Part model, mm, in its own coordinate system. A direction names the side the tool comes from. Round coordinates to 2 decimals unless told otherwise and drop trailing zeros. Loops run counter-clockwise (first coordinate to the right, second up) from the corner with the lowest first, then second, coordinate; pieces in that order, holes last.
from build123d import *

# Parameters (mm, degrees)
SKETCH1_R           = 1.5
BOSS_EXTRUDE2_DEPTH = 3.8
BOSS_EXTRUDE3_START = -3.8
SKETCH2_W           = 3.5
SKETCH2_H           = 7
SKETCH2_H_2         = 5.25
BOSS_EXTRUDE3_DEPTH = 3.8
CUT_EXTRUDE1_DEPTH  = 2.3
SKETCH4_W           = 3.5
SKETCH4_H           = 7
CUT_EXTRUDE2_DEPTH  = 1.5
FILLET1_R           = 4


with BuildPart() as part:
    # Sketch1 → Boss-Extrude2 (new body)
    # profile 1 of 5: a face of its own
    with BuildSketch(Plane(origin=(0, 0, 0), x_dir=(1, 0, 0), z_dir=(0, 1, 0))):
        with BuildLine():
            Line((-11.834936491, -1.25), (-11.834936491, 1.25))
            ThreePointArc((-11.834936491, 1.25), (-16.5, 0), (-11.834936491, -1.25))
        make_face()
        with Locations(Location((-14, 0, 0), (0, 0, 90))):
            Circle(SKETCH1_R, mode=Mode.SUBTRACT)
    # profile 2 of 5: a face of its own
    with BuildSketch(Plane(origin=(0, 0, 0), x_dir=(1, 0, 0), z_dir=(0, 1, 0))):
        with BuildLine():
            ThreePointArc((-11.5, 0), (-11.585185434, 0.647047613), (-11.834936491, 1.25))
            Line((-11.834936491, 1.25), (-11.834936491, -1.25))
            ThreePointArc((-11.834936491, -1.25), (-11.585185434, -0.647047613), (-11.5, 0))
        make_face()
    # profile 3 of 5: a face of its own
    with BuildSketch(Plane(origin=(0, 0, 0), x_dir=(1, 0, 0), z_dir=(0, 1, 0))):
        with BuildLine():
            Line((11.834936491, 1.25), (-11.834936491, 1.25))
            ThreePointArc((-11.834936491, 1.25), (-11.585185434, 0.647047613), (-11.5, 0))
            ThreePointArc((-11.5, 0), (-11.585185434, -0.647047613), (-11.834936491, -1.25))
            Line((-11.834936491, -1.25), (11.834936491, -1.25))
            ThreePointArc((11.834936491, -1.25), (11.5, 0), (11.834936491, 1.25))
        make_face()
    # profile 4 of 5: a face of its own
    with BuildSketch(Plane(origin=(0, 0, 0), x_dir=(1, 0, 0), z_dir=(0, 1, 0))):
        with BuildLine():
            Line((11.834936491, -1.25), (11.834936491, 1.25))
            ThreePointArc((11.834936491, 1.25), (11.5, 0), (11.834936491, -1.25))
        make_face()
    # profile 5 of 5: a face of its own
    with BuildSketch(Plane(origin=(0, 0, 0), x_dir=(1, 0, 0), z_dir=(0, 1, 0))):
        with BuildLine():
            ThreePointArc((16.5, 0), (14.647047613, 2.414814566), (11.834936491, 1.25))
            Line((11.834936491, 1.25), (11.834936491, -1.25))
            ThreePointArc((11.834936491, -1.25), (14.647047613, -2.414814566), (16.5, 0))
        make_face()
        with Locations(Location((14, 0, 0), (0, 0, 90))):
            Circle(SKETCH1_R, mode=Mode.SUBTRACT)
    extrude(amount=BOSS_EXTRUDE2_DEPTH)

    # Sketch2 → Boss-Extrude3 (add)
    with BuildSketch(Plane(origin=(0, 3.8, 0), x_dir=(1, 0, 0), z_dir=(0, 1, 0)).offset(BOSS_EXTRUDE3_START)):
        with Locations((-10.5, 10)):
            Rectangle(SKETCH2_W, SKETCH2_H)
        with BuildLine():
            Line((-8.75, 6.5), (-12.25, 6.5))
            Line((-12.25, 6.5), (-12.25, 1.785357107))
            ThreePointArc((-12.25, 1.785357107), (-12.024251438, 1.531802083), (-11.834936491, 1.25))
            Line((-11.834936491, 1.25), (-8.75, 1.25))
            Line((-8.75, 1.25), (-8.75, 6.5))
        make_face()
        with Locations((10.5, -3.875)):
            Rectangle(SKETCH2_W, SKETCH2_H_2)
        with Locations((10.5, -10)):
            Rectangle(SKETCH2_W, SKETCH2_H)
    extrude(amount=BOSS_EXTRUDE3_DEPTH)

    # Sketch3 → Cut-Extrude1 (cut)
    with BuildSketch(Plane.XZ):
        with BuildLine():
            Line((11.834936491, 1.25), (8.75, 1.25))
            Line((8.75, 1.25), (-11.834936491, 1.25))
            ThreePointArc((-11.834936491, 1.25), (-11.585185434, 0.647047613), (-11.5, 0))
            ThreePointArc((-11.5, 0), (-11.585185434, -0.647047613), (-11.834936491, -1.25))
            Line((-11.834936491, -1.25), (-8.75, -1.25))
            Line((-8.75, -1.25), (11.834936491, -1.25))
            ThreePointArc((11.834936491, -1.25), (11.5, 0), (11.834936491, 1.25))
        make_face()
        with BuildLine():
            Line((12.25, 6.5), (8.75, 6.5))
            Line((8.75, 6.5), (8.75, 1.25))
            Line((8.75, 1.25), (11.834936491, 1.25))
            ThreePointArc((11.834936491, 1.25), (12.024251438, 1.531802083), (12.25, 1.785357107))
            Line((12.25, 1.785357107), (12.25, 6.5))
        make_face()
        with BuildLine():
            ThreePointArc((-11.834936491, -1.25), (-12.024251438, -1.531802083), (-12.25, -1.785357107))
            Line((-12.25, -1.785357107), (-12.25, -6.5))
            Line((-12.25, -6.5), (-8.75, -6.5))
            Line((-8.75, -6.5), (-8.75, -1.25))
            Line((-8.75, -1.25), (-11.834936491, -1.25))
        make_face()
    extrude(amount=-CUT_EXTRUDE1_DEPTH, mode=Mode.SUBTRACT)

    # Sketch4 → Cut-Extrude2 (cut)
    with BuildSketch(Plane.XZ):
        with Locations((-10.5, -10)):
            Rectangle(SKETCH4_W, SKETCH4_H)
        with Locations((10.5, 10)):
            Rectangle(SKETCH4_W, SKETCH4_H)
    extrude(amount=-CUT_EXTRUDE2_DEPTH, mode=Mode.SUBTRACT)

    # Fillet1
    # the kernel refuses this fillet: 4 mm, written as the material it adds along each edge
    with BuildSketch(Plane(origin=(11.834936491, 2.3, -1.25), x_dir=(-1, 0, 0), z_dir=(0, 1, 0))) as fillet1_piece_1:
        with BuildLine():
            CenterArc((1.66736392, -4), FILLET1_R, 90, 36.128927472)
            ThreePointArc((-0.69105296, -0.769230769), (-0.305320518, -0.420735169), (0, 0))
            Line((0, 0), (1.66736392, 0))
        make_face()
    extrude(amount=1.5)
    with BuildSketch(Plane(origin=(-11.834936491, 2.3, 1.25), x_dir=(-0.668294067479168, 0, 0.743897196776644), z_dir=(0, 1, 0))) as fillet1_piece_2:
        with BuildLine():
            CenterArc((1.861299371, 3.913523616), FILLET1_R, 221.935536264, 36.128927472)
            Line((-1.114289416, 1.240347346), (0, 0))
            ThreePointArc((0, 0), (0.517027603, 0.05404774), (1.034055206, 0))
        make_face()
    extrude(amount=1.5)
    with BuildSketch(Plane(origin=(8.75, 2.3, 1.25), x_dir=(-1, 0, 0), z_dir=(0, 1, 0))) as fillet1_piece_3:
        with BuildLine():
            CenterArc((FILLET1_R, FILLET1_R), FILLET1_R, 180, 90)
            Line((0, FILLET1_R), (0, 0))
            Line((0, 0), (FILLET1_R, 0))
        make_face()
    extrude(amount=1.5)
    with BuildSketch(Plane(origin=(12.25, 3.8, 1.785357107), x_dir=(0.9778293887496555, 0, 0.20940316735301484), z_dir=(0, -1, 0))) as fillet1_piece_4:
        with BuildLine():
            CenterArc((4.81443119, 3.379568307), FILLET1_R, 167.912621371, 69.747753258)
            Line((0.903113635, 4.217180976), (0, 0))
            ThreePointArc((0, 0), (1.337341997, 0.387769808), (2.674683994, 0))
        make_face()
    extrude(amount=1.5)
    with BuildSketch(Plane(origin=(-12.25, 2.3, -1.785357107), x_dir=(-0.9778293887496644, 0, -0.20940316735297415), z_dir=(0, 1, 0))) as fillet1_piece_5:
        with BuildLine():
            CenterArc((4.81443119, -3.379568307), FILLET1_R, 122.339625371, 69.747753258)
            Line((0.903113635, -4.217180976), (0, 0))
            ThreePointArc((0, 0), (1.337341997, -0.387769808), (2.674683994, 0))
        make_face()
    extrude(amount=1.5)
    with BuildSketch(Plane(origin=(-8.75, 2.3, -1.25), x_dir=(0, 0, -1), z_dir=(0, 1, 0))) as fillet1_piece_6:
        with BuildLine():
            CenterArc((FILLET1_R, -FILLET1_R), FILLET1_R, 90, 90)
            Line((0, -FILLET1_R), (0, 0))
            Line((0, 0), (FILLET1_R, 0))
        make_face()
    extrude(amount=1.5)


solid = part.part
1) Slice it at A-A, the plane y = 3.2. Give the cut face in (x, z), then the cut area to 3 significant figures.
Values:
outline: (-14.87, -2.35) arc R4 cw to (-12.25, -6.1) - (-12.25, -13.5) - (-8.75, -13.5) - (-8.75, -5.25) arc R4 cw to (-4.75, -1.25) - (10.17, -1.25) arc R4 cw to (12.53, -2.02) arc R2.5 ccw (long way) to (14.87, 2.35) arc R4 cw to (12.25, 6.1) - (12.25, 13.5) - (8.75, 13.5) - (8.75, 5.25) arc R4 cw to (4.75, 1.25) - (-10.17, 1.25) arc R4 cw to (-12.53, 2.02) arc R2.5 ccw (long way) to start; hole circle Ø3 at (-14, 0); hole circle Ø3 at (14, 0)
area: 182 mm2
2) Tool access for faces 1 (the face through (7.609, 3.04, 2.453)), 2 (the face through (-11, 1.5, -10)), 3 (the face through (8.75, 3, 9)), 4 (the face through (12.25, 3, 10)), 5 (the face through (3, 3, -1.25)): list every direction of +Z, -Z, +X, -X, +Y, -Y with a clear straight run to the whole face (end or side of a thin tool).
Values:
face 1: +Z, +Y, -Y
face 2: -Z, +X, -X, -Y
face 3: +Z, -X, +Y, -Y
face 4: +Z, +X, +Y, -Y
face 5: -Z, +Y, -Y
3) Mould opens along X. For faces 6 (the face through (-12.25, 3, -10)), 7 (the face through (10, 3, 13.5)), 8 (the face through (-11.39, 3.04, 1.44)) say: released by +X, released by -X, zero draft, split by the parting line, or undercut.
Values:
face 6: released by -X
face 7: zero draft
face 8: undercut
4) Slice it at D-D, the plane z = 10.75. Give the cut face in (x, y).
Values:
outline: (8.75, 1.5) - (12.25, 1.5) - (12.25, 3.8) - (8.75, 3.8) - close
5) Wall check: line 1 along X through (y, z) = (2.4, 0); line 2 along X through (y, z) = (0.9, 0); line 3 along Z through (x, y) = (-14, 1.5). Give the ranges that are in metal, low to high.
Values:
line 1: x = -16.5 to -15.5, -12.5 to 12.5, 15.5 to 16.5
line 2: x = -16.5 to -15.5, -12.5 to -11.5, 11.5 to 12.5, 15.5 to 16.5
line 3: z = -2.5 to -1.5, 1.5 to 2.5
6) Slice it at B-B, the plane y = 1.1. Give the cut face in (x, z), then the cut area to 3 significant figures.
Values:
outline: circle Ø5 at (-14, 0); circle Ø5 at (14, 0); hole circle Ø3 at (-14, 0); hole circle Ø3 at (14, 0)
area: 25.1 mm2
7) Slice it at C-C, the plane x = 14. Give the cut face in (y, z).
Values:
outline: (0, -2.5) - (3.8, -2.5) - (3.8, -1.5) - (0, -1.5) - close; (0, 1.5) - (3.8, 1.5) - (3.8, 2.79) - (2.3, 2.79) - (2.3, 2.5) - (0, 2.5) - close
8) Drop flat-ended pins along their axis: pin 1 Ø6.5 at (x, z) = (-3.5, 1) entering from -Y; pin 2 Ø1.2 at (y, z) = (2, 7.5) entering from -X; pin 3 Ø4 at (x, z) = (10.5, 10.5) entering from -Y. Give the stop position or say it passes through.
Values:
pin 1: stops at y = 2.3
pin 2: stops at x = 8.75
pin 3: stops at y = 1.5
